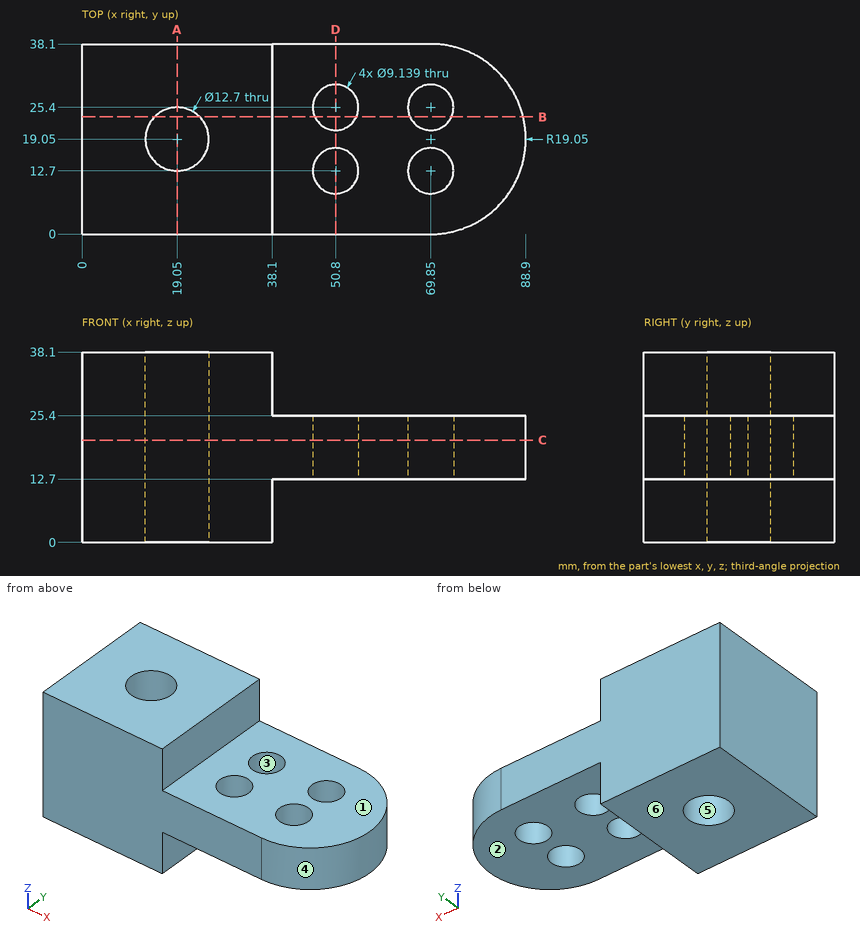
Here's the drawing with two shaded views (mm, measured from the low corner). I have some questions. A direction names the side the tool comes from. Round coordinates to 2 decimals unless told otherwise and drop trailing zeros. Loops run counter-clockwise (first coordinate to the right, second up) from the corner with the lowest first, then second, coordinate; pieces in that order, holes last. Notation, with made-up numbers: M -10,-24 L 45,-24 A16 cw 45,-20 Z; hole C 84.25,-2.5 d5. An arc over 180 degrees is marked long. Put each result on its own line as item: value.
Q1. Imagine slicing it at A-A (x = 19.05). Write out the boundary of the cut face in (y, z), then the cut area to 3 significant figures.
Check result:
outline: M 0,0 L 12.7,0 L 12.7,38.1 L 0,38.1 Z; M 25.4,0 L 38.1,0 L 38.1,38.1 L 25.4,38.1 Z
area: 968 mm2
Q2. Imagine slicing it at D-D (x = 50.8). Write out the boundary of the cut face in (y, z).
Check result:
outline: M 0,12.7 L 8.13,12.7 L 8.13,25.4 L 0,25.4 Z; M 17.27,12.7 L 20.83,12.7 L 20.83,25.4 L 17.27,25.4 Z; M 29.97,12.7 L 38.1,12.7 L 38.1,25.4 L 29.97,25.4 Z
Q3. Imagine slicing it at C-C (z = 20.5). Write out the boundary of the cut face in (x, y).
Check result:
outline: M 0,0 L 69.85,0 A19.05 ccw 69.85,38.1 L 0,38.1 Z; hole C 19.05,19.05 d12.7; hole C 50.8,12.7 d9.14; hole C 50.8,25.4 d9.14; hole C 69.85,12.7 d9.14; hole C 69.85,25.4 d9.14
Q4. Thinking about a two-plate mould opening in Y: for the marked faces 4, 5 and 6, which applies, released by +Y, released by -Y, zero draft, split by the parting line, or undercut?
Check result:
face 4: split by the parting line
face 5: undercut
face 6: zero draft
Q5. For pin 1 (14.5 mm diameter, centred on x = 50.8, y = 25.4, fed in from +Z); pin 2 (19 mm diameter, centred on x = 72.5, y = 19, fed in from -Z); pin 3 (1 mm diameter, centred on y = 24, z = 29.5, fed in from +X), each with a flat end and sliding along its axis, tell me the tip position at first contact or that it passes through.
Check result:
pin 1: z = 25.4
pin 2: z = 12.7
pin 3: x = 38.1
Q6. I need wall thicknesses on probe 1 along Y at (x, z) = (50.8, 18.5); probe 2 along X at (y, z) = (28, 24.5); probe 3 along X at (y, z) = (10.5, 22.5) (1 decimal). Which ranges of each line are inside material? Lowest first, please.
Check result:
probe 1: 0 to 8.13, 17.27 to 20.83, 29.97 to 38.1
probe 2: 0 to 47.04, 54.56 to 66.09, 73.61 to 86.67
probe 3: 0 to 46.8, 54.8 to 65.8, 73.9 to 86.9
Q7. Imagine slicing it at B-B (y = 23.5). Write out the boundary of the cut face in (x, z), then the cut area to 3 significant figures.
Check result:
outline: M 0,0 L 14.52,0 L 14.52,38.1 L 0,38.1 Z; M 23.58,0 L 38.1,0 L 38.1,12.7 L 46.64,12.7 L 46.64,25.4 L 38.1,25.4 L 38.1,38.1 L 23.58,38.1 Z; M 54.96,12.7 L 65.69,12.7 L 65.69,25.4 L 54.96,25.4 Z; M 74.01,12.7 L 88.37,12.7 L 88.37,25.4 L 74.01,25.4 Z
area: 1,530 mm2
Q8. On a 3-axis mill with a long thin cutter (end or side, diameter ignored), from which of +Z, -Z, +X, -X, +Y, -Y can I reach the whole of each face in a straight line? I mean the marked faces 1, 2 and 3. Say none if no direction works.
Check result:
face 1: +Z, +X, +Y, -Y
face 2: -Z, +X, +Y, -Y
face 3: +Z, -Z
